The model under review builds one solid part; all positions refer to its coordinate system, in mm. Face numbers are marked on the shaded views. A direction names the side the tool comes from. Round coordinates to 2 decimals unless told otherwise and drop trailing zeros. Loops run counter-clockwise (first coordinate to the right, second up) from the corner with the lowest first, then second, coordinate; pieces in that order, holes last. Notation, with made-up numbers: M 25.5,40.25 L 48.5,40.25 A27 ccw 48.5,75.25 Z; hole C -26.5,28 d3. An arc over 180 degrees is marked long. One line per question, with ' | ' between items.
from build123d import *

# Parameters (mm, degrees)
SKETCH_2_R          = 25
SKETCH_2_R_2        = 1.55
EXTRUDE_1_DEPTH     = 3
SKETCH_3_R          = 12.5
EXTRUDE_2_DEPTH     = 30
SKETCH_4_R          = 4
CUT_EXTRUDE_1_DEPTH = 18
SKETCH_5_R          = 2.467025672
SKETCH_5_R_2        = 1.5
CUT_EXTRUDE_2_DEPTH = 33
SKETCH_6_R          = 10.5
CUT_EXTRUDE_3_DEPTH = 1
FILLET_1_R          = 2
SKETCH_8_R          = 9.571067812
EXTRUDE_4_DEPTH     = 18
SKETCH_9_R          = 3.5
SKETCH_9_R_2        = 3
CUT_EXTRUDE_7_DEPTH = 20
SKETCH_10_R         = 2.467025672
SKETCH_10_R_2       = 1.55
EXTRUDE_5_DEPTH     = 12


with BuildPart() as part:
    # 草图2 → 凸台-拉伸1 (new body)
    with BuildSketch(Plane.XY.offset(0.048295154)):
        with Locations((-1.050726952, -17)):
            Circle(SKETCH_2_R)
        with Locations((-14.75, -3)):
            Circle(SKETCH_2_R_2, mode=Mode.SUBTRACT)
        with Locations((-14.75, -17)):
            Circle(SKETCH_2_R_2, mode=Mode.SUBTRACT)
        with Locations((-14.75, -31)):
            Circle(SKETCH_2_R_2, mode=Mode.SUBTRACT)
        with Locations((15.5, -23.95)):
            Circle(SKETCH_2_R_2, mode=Mode.SUBTRACT)
        with Locations((15.5, -9.95)):
            Circle(SKETCH_2_R_2, mode=Mode.SUBTRACT)
    extrude(amount=EXTRUDE_1_DEPTH)

    # 草图3 → 凸台-拉伸2 (add)
    with BuildSketch(Plane.XY.offset(3.048295154)):
        with Locations(Location((-1.050726952, -17, 0), (0, 0, 184.300454135))):
            Circle(SKETCH_3_R)
    extrude(amount=EXTRUDE_2_DEPTH)

    # 草图4 → 切除-拉伸1 (cut)
    with BuildSketch(Plane(origin=(0, 0, 0.048295154), x_dir=(-1, 0, 0), z_dir=(0, 0, -1))):
        with BuildLine():
            ThreePointArc((8.550726952, -12), (6.050726952, -9.5), (3.550726952, -12))
            Line((3.550726952, -12), (6.050726952, -12))
            Line((6.050726952, -12), (6.050726952, -14.5))
            ThreePointArc((6.050726952, -14.5), (7.818493905, -13.767766953), (8.550726952, -12))
        make_face()
        with BuildLine():
            Line((6.050726952, -12), (3.550726952, -12))
            ThreePointArc((3.550726952, -12), (4.282959999, -13.767766953), (6.050726952, -14.5))
            Line((6.050726952, -14.5), (6.050726952, -12))
        make_face()
        with BuildLine():
            ThreePointArc((8.550726952, -22), (7.818493905, -20.232233047), (6.050726952, -19.5))
            Line((6.050726952, -19.5), (6.050726952, -22))
            Line((6.050726952, -22), (3.550726952, -22))
            ThreePointArc((3.550726952, -22), (6.050726952, -24.5), (8.550726952, -22))
        make_face()
        with BuildLine():
            Line((6.050726952, -22), (6.050726952, -19.5))
            ThreePointArc((6.050726952, -19.5), (4.282959999, -20.232233047), (3.550726952, -22))
            Line((3.550726952, -22), (6.050726952, -22))
        make_face()
        with BuildLine():
            ThreePointArc((-1.449273048, -22), (-2.181506095, -20.232233047), (-3.949273048, -19.5))
            Line((-3.949273048, -19.5), (-3.949273048, -22))
            Line((-3.949273048, -22), (-1.449273048, -22))
        make_face()
        with BuildLine():
            Line((-3.949273048, -22), (-3.949273048, -19.5))
            ThreePointArc((-3.949273048, -19.5), (-5.717040001, -23.767766953), (-1.449273048, -22))
            Line((-1.449273048, -22), (-3.949273048, -22))
        make_face()
        with BuildLine():
            Line((-3.949273048, -14.5), (-3.949273048, -12))
            Line((-3.949273048, -12), (-1.449273048, -12))
            ThreePointArc((-1.449273048, -12), (-5.717040001, -10.232233047), (-3.949273048, -14.5))
        make_face()
        with BuildLine():
            Line((-1.449273048, -12), (-3.949273048, -12))
            Line((-3.949273048, -12), (-3.949273048, -14.5))
            ThreePointArc((-3.949273048, -14.5), (-2.181506095, -13.767766953), (-1.449273048, -12))
        make_face()
        with Locations((1.050726952, -17)):
            Circle(SKETCH_4_R)
    extrude(amount=-CUT_EXTRUDE_1_DEPTH, mode=Mode.SUBTRACT)

    # 草图5 → 切除-拉伸2 (cut)
    with BuildSketch(Plane(origin=(0, 0, 0.048295154), x_dir=(-1, 0, 0), z_dir=(0, 0, -1))):
        with Locations((1.050726952, -17)):
            Circle(SKETCH_5_R)
        with Locations((6.050726952, -12)):
            Circle(SKETCH_5_R_2)
        with Locations((-3.949273048, -12)):
            Circle(SKETCH_5_R_2)
        with Locations((-3.949273048, -22)):
            Circle(SKETCH_5_R_2)
        with Locations((6.050726952, -22)):
            Circle(SKETCH_5_R_2)
    extrude(amount=-CUT_EXTRUDE_2_DEPTH, mode=Mode.SUBTRACT)

    # 草图6 → 切除-拉伸3 (cut)
    with BuildSketch(Plane.XY.offset(33.048295154)):
        with Locations((-1.050726952, -17)):
            Circle(SKETCH_6_R)
    extrude(amount=-CUT_EXTRUDE_3_DEPTH, mode=Mode.SUBTRACT)

    # 圆角1
    # the kernel refuses this fillet: 2 mm, written as the material it adds along each edge
    with BuildSketch(Plane(origin=(-1.050726952, -17, 3.048295154), x_dir=(-0.9999950652018734, -0.0031415874810074846, 0), z_dir=(-0.0031415874810074846, 0.9999950652018734, 0))) as fillet_1_piece_1_section:
        with BuildLine():
            CenterArc((12.5 + FILLET_1_R, FILLET_1_R), FILLET_1_R, 180, 90)
            Line((12.5, FILLET_1_R), (12.5, 0))
            Line((12.5, 0), (12.5 + FILLET_1_R, 0))
        make_face()
    fillet_1_piece_1 = revolve(axis=Axis((-1.050726952, -17, 3.048295154), (0, 0, 1)), revolution_arc=359.64, mode=Mode.PRIVATE)
    fillet_1_piece_1 = fillet_1_piece_1 - Plane(origin=(-14.75, -17, 3.605266613), x_dir=(1, 0, 0), z_dir=(0, 0, -1)) * Cylinder(1.55, 59, mode=Mode.PRIVATE)
    add(fillet_1_piece_1)

    # 草图8 → 凸台-拉伸4 (add)
    with BuildSketch(Plane(origin=(0, 0, 0.048295154), x_dir=(-1, 0, 0), z_dir=(0, 0, -1))):
        with Locations((1.050726952, -17)):
            Circle(SKETCH_8_R)
    extrude(amount=-EXTRUDE_4_DEPTH)

    # 草图9 → 切除-拉伸7 (cut)
    with BuildSketch(Plane(origin=(0, 0, 0.048295154), x_dir=(-1, 0, 0), z_dir=(0, 0, -1))):
        with BuildLine():
            ThreePointArc((-0.949273048, -12), (-6.070593392, -9.878679656), (-3.949273048, -15))
            Line((-3.949273048, -15), (-3.949273048, -12))
            Line((-3.949273048, -12), (-0.949273048, -12))
        make_face()
        with BuildLine():
            Line((-3.949273048, -12), (-3.949273048, -15))
            ThreePointArc((-3.949273048, -15), (-1.827952704, -14.121320344), (-0.949273048, -12))
            Line((-0.949273048, -12), (-3.949273048, -12))
        make_face()
        with Locations((1.050726952, -17)):
            Circle(SKETCH_9_R)
        with Locations((6.050726952, -12)):
            Circle(SKETCH_9_R_2)
        with Locations((6.050726952, -22)):
            Circle(SKETCH_9_R_2)
        with Locations((-3.949273048, -22)):
            Circle(SKETCH_9_R_2)
    extrude(amount=-CUT_EXTRUDE_7_DEPTH, mode=Mode.SUBTRACT)

    # 草图10 → 凸台-拉伸5 (add)
    with BuildSketch(Plane(origin=(0, 0, 20.048295154), x_dir=(-1, 0, 0), z_dir=(0, 0, -1))):
        with Locations((1.050726952, -17)):
            Circle(SKETCH_10_R)
        with Locations((1.050726952, -17)):
            Circle(SKETCH_10_R_2, mode=Mode.SUBTRACT)
    extrude(amount=-EXTRUDE_5_DEPTH)


solid = part.part
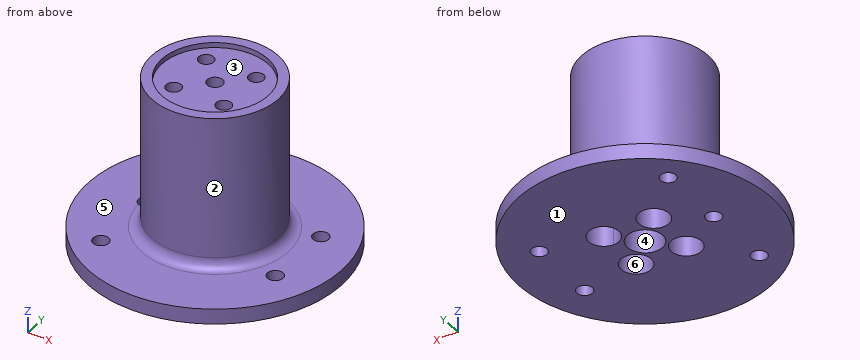
1) Add section A-A on y = -17. State the section outline as (x, z) points, then the cut area to 3 significant figures.
Output values:
outline: M -26.05,0.05 L -16.3,0.05 L -16.3,3.05 L -26.05,3.05 Z; M -13.55,3.05 L -13.2,3.05 L -13.2,0.05 L -4.55,0.05 L -4.55,20.05 L -2.6,20.05 L -2.6,32.05 L -11.55,32.05 L -11.55,33.05 L -13.55,33.05 Z; M 0.5,20.05 L 2.45,20.05 L 2.45,0.05 L 23.95,0.05 L 23.95,3.05 L 13.45,3.05 A2 cw 11.45,5.05 L 11.45,33.05 L 9.45,33.05 L 9.45,32.05 L 0.5,32.05 Z | area: 693 mm²
2) Add section C-C on x = -14.75. State how many separate pieces and enclosed holes the cut face has, then the cut area to 3 significant figures.
Output values:
separate pieces: 4 | enclosed holes: 0 | area: 97.9 mm²
3) For line 1 (Y direction, x = -5, z = 6.5); line 2 (Y direction, x = -5, z = 24); line 3 (X direction, y = -13, z = 27), list the stretches that pass through material, from the lowest coordinate up.
Output values:
line 1: y = -28.86 to -24.81, -19.19 to -14.81, -9.19 to -5.14 | line 2: y = -28.86 to -23.07, -20.93 to -13.07, -10.93 to -5.14 | line 3: x = -12.89 to -7.17, -4.93 to 2.83, 5.07 to 10.79
4) Insertion check: P1, Ø8, axis at x = -4, z = 3.5, coming from the +Y side; P2, Ø6.5, axis at x = -4.5, y = -12, coming from the -Z side; P3, Ø1, axis at x = -21, y = -14.5, coming from the +Z side; P4, Ø3.5, axis at x = 3.95, y = -12, coming from the +Z side. Each pin has a flat end and moves straight along its axis. Give the tip position at first contact, or say it passes through.
Output values:
P1: stops at y = 8 | P2: stops at z = 0.05 | P3: stops at z = 3.05 | P4: stops at z = 32.05
5) Add section D-D on y = 5. State the section outline as (x, z) points, then the cut area to 3 significant figures.
Output values:
outline: M -12.93,0.05 L 10.82,0.05 L 10.82,3.05 L -12.93,3.05 Z | area: 71.2 mm²
6) Mouldability with a two-part tool opening along X and no side actions: class the marked faces 1, 2, 3 and 4 as +X half, -X half, draft (parallel to the pull), parting line (faces both ways), or undercut.
Output values:
face 1: draft | face 2: parting line | face 3: undercut | face 4: undercut
7) Machinability: for the marked faces 5 and 6, which of the approach directions +Z, -Z, +X, -X, +Y, -Y give a long, thin tool a straight path to every point of the face, cutting with its end or side? Answer none if there is none.
Output values:
face 5: +Z | face 6: -Z
8) Add section B-B on z = 17. State the section outline as (x, y) points.
Output values:
outline: C -1.05,-17 d25; hole C -6.05,-22 d6; hole C -6.05,-12 d6; hole C -1.05,-17 d7; hole C 3.95,-22 d6; hole C 3.95,-12 d6
